Build history of the part. All positions in model axes, mm. Give positions to 0.01 mm unless a question says otherwise; leave off trailing zeros. Order: outer loops, then holes, each group sorted by start corner. A loop starts at its lowest first (then second) coordinate and runs counter-clockwise, first axis right, second up. Notation, with made-up numbers: M -3.5,64 L 7.5,64 A18 ccw 7.5,79 Z; hole C 27,-34.75 d8. An arc over 180 degrees is marked long. One line per item, written item: value.
Autodesk Inventor part; units mm, degrees
ref_plane "YZ Plane" through (0, 0, 0) normal (1, 0, 0) x (0, 1, 0)
ref_plane "XZ Plane" through (0, 0, 0) normal (0, 1, 0) x (-1, 0, 0)
ref_plane "XY Plane" through (0, 0, 0) normal (0, 0, 1) x (1, 0, 0)
sketch "Sketch1" plane through (0, 0, 0) normal (0, 1, 0) x (-1, 0, 0)
  line L0 (0, 0) -> (200, 0)
  line L1 (200, 0) -> (200, -200)
  line L2 (200, -200) -> (0, -200)
  line L3 (0, -200) -> (0, 0)
  dimension "d0" = 200
  dimension "d1" = 200
extrude "Extrusion1" add sketch "Sketch1" along normal blind 4
sketch "Sketch2" plane through (0, 4, 0) normal (0, 1, 0) x (1, 0, 0)
  circle A0 centre (-197, 197) radius 1.5
  line L0 (0, 200) -> (-200, 200)
  line L1 (-200, 200) -> (-200, 0)
  circle A1 centre (-197, 3) radius 1.5
  line L2 (-200, 0) -> (0, 0)
  circle A2 centre (-3, 197) radius 1.5
  line L3 (0, 0) -> (0, 200)
  circle A3 centre (-3, 3) radius 1.5
  dimension "d4" = 3
  dimension "d5" = 3
  dimension "d6" = 3
  dimension "d7" = 3
  dimension "d8" = 3
  dimension "d9" = 3
  dimension "d10" = 3
  dimension "d11" = 3
  dimension "d12" = 3
  dimension "d13" = 3
  dimension "d14" = 3
  dimension "d15" = 3
hole "Hole1" at (-197, 4, -197) at (-3, 4, -197) at (-197, 4, -3) at (-3, 4, -3) direction (0, -1, 0) diameter 3 end through all
sketch "Sketch3" plane through (0, 4, 0) normal (0, 1, 0) x (1, 0, 0)
  circle A0 centre (-65, 65) radius 40
  line L0 (0, 0) -> (0, 200)
  line L1 (-200, 0) -> (0, 0)
  circle A1 centre (-140, 140) radius 37.5
  line L2 (0, 200) -> (-200, 200)
  line L3 (-200, 200) -> (-200, 0)
  circle A2 centre (-140, 140) radius 55
  line L4 (-185, 78) -> (-135, 78)
  line L5 (-135, 78) -> (-135, 10)
  line L6 (-135, 10) -> (-185, 10)
  line L7 (-185, 10) -> (-185, 78)
  circle A3 centre (-65, 65) radius 50
  circle A4 centre (-65, 65) radius 60
  line L8 (-185, 19) -> (-135, 19)
  line L9 (-135, 19) -> (-135, 69)
  line L10 (-135, 69) -> (-185, 69)
  line L11 (-185, 69) -> (-185, 19)
  dimension "d23" = 80
  dimension "d24" = 65
  dimension "d25" = 65
  dimension "d26" = 75
  dimension "d29" = 140
  dimension "d30" = 140
  dimension "d31" = 110
  dimension "d32" = 50
  dimension "d33" = 68
  dimension "d34" = 10
  dimension "d59" = 100
  dimension "d60" = 120
  dimension "d61" = 135
  dimension "d62" = 50
  dimension "d63" = 50
  dimension "d64" = 9
extrude "Extrusion2" cut sketch "Sketch3" against normal through all contours A0 | A1 | L10 L5 L8 L7
sketch "Sketch4" plane through (0, 4, 0) normal (0, 1, 0) x (1, 0, 0)
  circle A0 centre (-140, 140) radius 37.5
  circle A1 centre (-140, 140) radius 47.5
  circle A2 centre (-140, 187.5) radius 2
  circle A3 centre (-187.5, 140) radius 2
  circle A4 centre (-140, 92.5) radius 2
  circle A5 centre (-92.5, 140) radius 2
  point P0 (0, 0)
  dimension "d38" = 95
  dimension "d39" = 4
  dimension "d42" = 360
hole "Hole2" at (-187.5, 4, -140) at (-140, 4, -92.5) at (-140, 4, -187.5) at (-92.5, 4, -140) direction (0, -1, 0) diameter 4 end through all countersink diameter 8 countersink angle 90
thread "Thread1"
thread "Thread2"
thread "Thread3"
thread "Thread4"
thread "Thread5"
thread "Thread6"
thread "Thread7"
thread "Thread8"
fillet "Fillet1" radius 2 4 edges at (-185, 2, -69) (-185, 2, -19) (-135, 2, -69) (-135, 2, -19)
properties part number "Housing_lid" material "Aluminum 6061"
1) Pin check, flat tip, straight feed: pin 1 (5 mm diameter, centred on x = -187.5, z = -140, fed in from +Y). Stop position of the tip, or through.
Check values:
pin 1: y = 2.5
2) Saw through at D-D, the plane z = -170. Write the cut outline in (x, y), then the cut area to 3 significant figures.
Check values:
outline: M -200,0 L -162.5,0 L -162.5,4 L -200,4 Z; M -117.5,0 L 0,0 L 0,4 L -117.5,4 Z
area: 620 mm^2
3) Saw through at C-C, the plane y = 2.9. Give the number of separate pieces and of enclosed holes in the cut face, then the cut area to 3 significant figures.
Check values:
separate pieces: 1
enclosed holes: 11
area: 27,900 mm^2
4) Saw through at A-A, the plane x = -65. Write the cut outline in (y, z).
Check values:
outline: M 0,-200 L 4,-200 L 4,-105 L 0,-105 Z; M 0,-25 L 4,-25 L 4,0 L 0,0 Z
5) Saw through at B-B, the plane z = -33. Write the cut outline in (x, y), then the cut area to 3 significant figures.
Check values:
outline: M -200,0 L -185,0 L -185,4 L -200,4 Z; M -135,0 L -89,0 L -89,4 L -135,4 Z; M -41,0 L 0,0 L 0,4 L -41,4 Z
area: 408 mm^2
6) Mould opens along Z. For faces 1 (the face through (-141.293, 2.125, -189.186)), 2 (the face through (-99, 4, -99)) say: released by +Z, released by -Z, zero draft, split by the parting line, or undercut.
Check values:
face 1: undercut
face 2: zero draft
7) Drill centre lines: probe 1 along X at (y, z) = (1.4, -140); probe 2 along Z at (x, y) = (-3, 3.2); probe 3 along X at (y, z) = (2.5, -65). Where is each one in solid material? Low to high. Write a range as from..to.
Check values:
probe 1: -200..-189.5, -185.5..-177.5, -102.5..-94.5, -90.5..0
probe 2: -200..-198.5, -195.5..-4.5, -1.5..0
probe 3: -200..-185, -135..-105, -25..0
